Geometry check sheet. Reference: drawing and pictorial views, mm from the part's lowest x, y, z. A direction names the side the tool comes from. Give positions to 0.01 mm unless a question says otherwise; leave off trailing zeros. Order: outer loops, then holes, each group sorted by start corner. A loop starts at its lowest first (then second) coordinate and runs counter-clockwise, first axis right, second up.
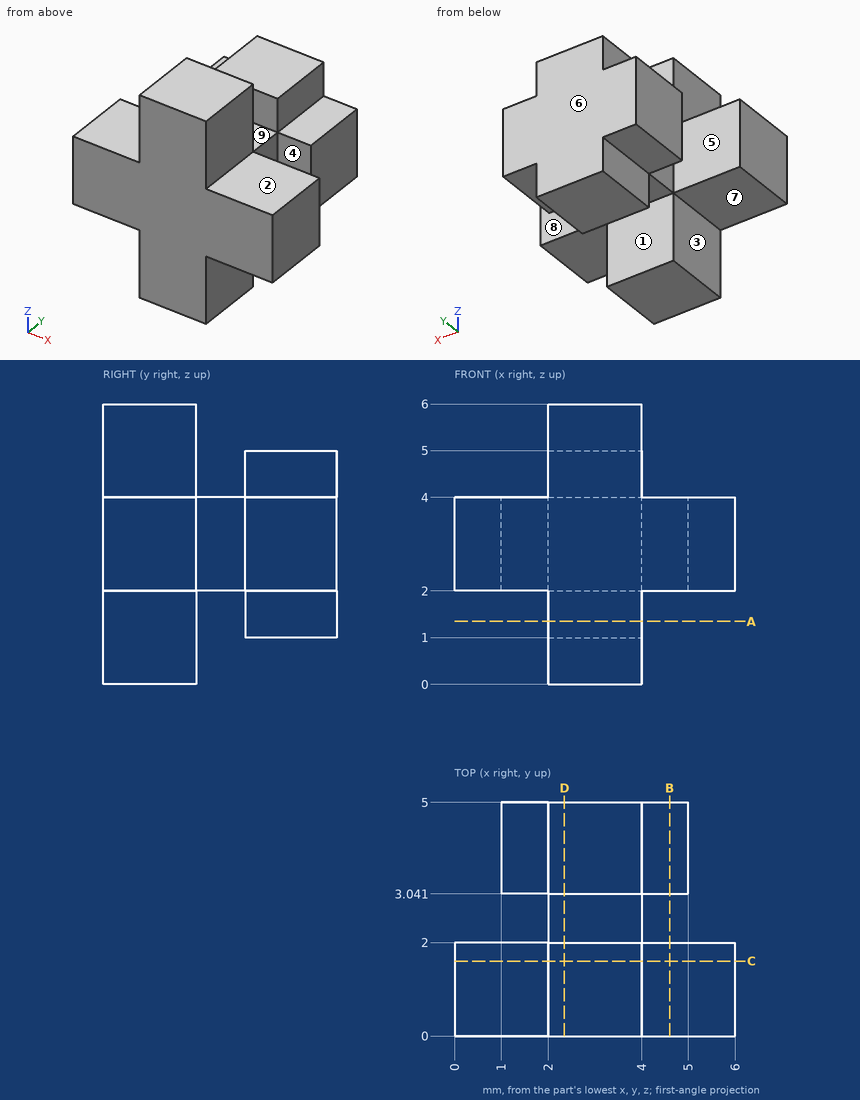
(1) Gauge pin test, flat ends, axial feed: pin 1 Ø2 at (x, y) = (0.5, 1) entering from -Z; pin 2 Ø1 at (y, z) = (4, 3) entering from +X; pin 3 Ø1.1 at (x, y) = (4.5, 3.5) entering from -Z. Record the tip position at first contact, or that the pin passes through.
Response values:
pin 1: stops at z = 2
pin 2: stops at x = 5
pin 3: stops at z = 1
(2) Cross-section at C-C on y = 1.6. Enter the section's corners in (x, z), then the cut area to 3 significant figures.
Response values:
outline: (0, 2) - (2, 2) - (2, 0) - (4, 0) - (4, 2) - (6, 2) - (6, 4) - (4, 4) - (4, 6) - (2, 6) - (2, 4) - (0, 4) - close
area: 20.0 mm2
(3) Release check for a two-part mould opening along Y. For the marked faces 6, 7, 8 and 9 record: released by +Y, released by -Y, zero draft, split by the parting line, or undercut.
Response values:
face 6: released by +Y
face 7: zero draft
face 8: undercut
face 9: undercut
(4) Set-up check for the marked faces 1, 2, 3, 4 and 5: record each of +Z, -Z, +X, -X, +Y, -Y from which the full face is reachable in a straight line by a thin tool's end or side.
Response values:
face 1: -Z, +X, -X
face 2: +Z, +X, +Y, -Y
face 3: -Z, -X, +Y, -Y
face 4: +Z, -Z, +X
face 5: +Z, -Z, -X
(5) Cross-section at D-D on x = 2.35. Enter the section's corners in (y, z), then the cut area to 3 significant figures.
Response values:
outline: (0, 0) - (2, 0) - (2, 2) - (3.04, 2) - (3.04, 1) - (5, 1) - (5, 5) - (3.04, 5) - (3.04, 4) - (2, 4) - (2, 6) - (0, 6) - close
area: 21.9 mm2
(6) Cross-section at A-A on z = 1.35. Enter the section's corners in (x, y).
Response values:
outline: (2, 0) - (4, 0) - (4, 2) - (2, 2) - close; (2, 3.04) - (4, 3.04) - (4, 5) - (2, 5) - close
(7) Cross-section at B-B on x = 4.6. Enter the section's corners in (y, z).
Response values:
outline: (0, 2) - (2, 2) - (2, 4) - (0, 4) - close; (3.04, 2) - (5, 2) - (5, 4) - (3.04, 4) - close
(8) Material ranges on L1, parallel to Z at x = 1.4, y = 3.85; L2, parallel to Z at x = 3.1, y = 4.55, recorded low to high.
Response values:
L1: z = 2 to 4
L2: z = 1 to 5
